For this review, take the finished solid that the model builds, in its own axes (mm). A direction names the side the tool comes from. Coordinates: 2 decimals unless noted, no trailing zeros. Write each loop counter-clockwise with the first axis right and the second up, starting at its lowest first coordinate (ties: lowest second). Pieces come first, ordered by that corner, then holes.
1) Mouldability with a two-part tool opening along Y and no side actions: class faces 1 (the face through (0, 60, 3)), 2 (the face through (-18.359, 4.203, 4.028)), 3 (the face through (12, 32, 6)) as pulls with the +Y half, pulls with the -Y half, needs draft (parallel to the pull), parting line crosses it, or undercut.
2) We need section B-B on z = 3.6. Write out the cut boundary in (x, y), then the cut area to 3 significant figures.
3) We need section C-C on y = 54. Write out the cut boundary in (x, z), then the cut area to 3 significant figures.
4) We need section D-D on y = 14.5. Write out the cut boundary in (x, z).
5) Insertion check: P1, Ø1.5, axis at x = 11.5, y = 27, coming from the +Z side. The pin has a flat end and moves straight along its axis. Give the tip position at first contact, or say it passes through.
6) We need section A-A on x = 0. Write out the cut boundary in (y, z), then the cut area to 3 significant figures.
7) To check wall thickness, follow line 1 along Z through (x, y) = (-8, 12.5); line 2 along X through (y, z) = (54, 4.6); line 3 along Y through (x, z) = (-1.5, 1.65). State the ranges of each line that lie inside material, in increasing order.
8) For faces 4 (the face through (0, 24, 0)), 5 (the face through (19.5, 8, 4)), list the 3-axis set-ups (+Z, -Z, +X, -X, +Y, -Y) from which the entire face can be reached by the end or side of a thin tool; tool diameter is ignored.
Autodesk Inventor part; units mm, degrees
ref_plane "YZ Plane" through (0, 0, 0) normal (1, 0, 0) x (0, 1, 0)
ref_plane "XZ Plane" through (0, 0, 0) normal (0, 1, 0) x (-1, 0, 0)
ref_plane "XY Plane" through (0, 0, 0) normal (0, 0, 1) x (1, 0, 0)
sketch "Sketch1" plane through (0, 0, 0) normal (0, 0, 1) x (1, 0, 0)
  line L0 (-22.5, 0) -> (22.5, 0)
  line L1 (22.5, 0) -> (22.5, 10)
  line L2 (22.5, 10) -> (5.6342, 56.0629)
  arc A0 (5.6342, 56.0629) -> (-5.6342, 56.0629) centre (0, 54) ccw
  line L3 (-5.6342, 56.0629) -> (-22.5, 10)
  line L4 (-22.5, 10) -> (-22.5, 0)
  point P0 (0, 0)
  point P1 (0, 0)
  dimension "d0" = 45
  dimension "d1" = 10
  dimension "d2" = 6
  dimension "d3" = 54
extrude "Extrusion1" add sketch "Sketch1" along normal blind 6
sketch "Sketch2" plane through (0, 0, 6) normal (0, 0, 1) x (1, 0, 0)
  line L0 (22.5, 0) -> (22.5, 10)
  line L1 (22.5, 10) -> (5.6342, 56.0629)
  line L2 (-5.6342, 56.0629) -> (-22.5, 10)
  line L3 (-22.5, 10) -> (-22.5, 0)
  line L4 (-22.5, 0) -> (22.5, 0)
  line L5 (-19.5, 9.468) -> (-7.5123, 42.2083)
  line L6 (7.5123, 42.2083) -> (19.5, 9.468)
  line L7 (19.5, 9.468) -> (19.5, 7)
  line L8 (15.5, 3) -> (-15.5, 3)
  line L9 (-19.5, 7) -> (-19.5, 9.468)
  arc A0 (7.5123, 42.2083) -> (-7.5123, 42.2083) centre (0, 39.4577) ccw
  arc A1 (-19.5, 7) -> (-15.5, 3) centre (-15.5, 7) ccw
  arc A2 (15.5, 3) -> (19.5, 7) centre (15.5, 7) ccw
  point P0 (0, 0)
  dimension "d6" = 3
  dimension "d7" = 8
  dimension "d8" = 3
  dimension "d9" = 4
extrude "Extrusion2" cut sketch "Sketch2" against normal blind 4
sketch "Sketch3" plane through (0, 0, 6) normal (0, 0, 1) x (1, 0, 0)
  arc A0 (5.6342, 56.0629) -> (-5.6342, 56.0629) centre (0, 54) ccw
  point P0 (0, 0)
hole "Hole1" at (0, 54, 6) direction (0, 0, -1) diameter 6 end through all
properties part number "Bearing Short" material "Steel"
Result:
1. face 1: pulls with the +Y half
1. face 2: undercut
1. face 3: needs draft
2. outline: (-22.5, 0) - (22.5, 0) - (22.5, 10) - (5.63, 56.06) arc R6 ccw to (-5.63, 56.06) - (-22.5, 10) - close; hole (-19.5, 7) arc R4 ccw to (-15.5, 3) - (15.5, 3) arc R4 ccw to (19.5, 7) - (19.5, 9.47) - (7.51, 42.21) arc R8 ccw to (-7.51, 42.21) - (-19.5, 9.47) - close; hole circle Ø6 at (0, 54)
2. area: 563 mm2
3. outline: (-6.39, 0) - (-3, 0) - (-3, 6) - (-6.39, 6) - close; (3, 0) - (6.39, 0) - (6.39, 6) - (3, 6) - close
3. area: 40.7 mm2
4. outline: (-20.85, 0) - (20.85, 0) - (20.85, 6) - (17.66, 6) - (17.66, 2) - (-17.66, 2) - (-17.66, 6) - (-20.85, 6) - close
5. P1: stops at z = 2
6. outline: (0, 0) - (51, 0) - (51, 6) - (47.46, 6) - (47.46, 2) - (3, 2) - (3, 6) - (0, 6) - close; (57, 0) - (60, 0) - (60, 6) - (57, 6) - close
6. area: 146 mm2
7. line 1: z = 0 to 2
7. line 2: x = -6.39 to -3, 3 to 6.39
7. line 3: y = 0 to 51.4, 56.6 to 59.81
8. face 4: -Z, +X, -X, +Y, -Y
8. face 5: +Z
